Work out the finished part from the listing and answer in its coordinate system (mm). Face numbers are marked on the shaded views. A direction names the side the tool comes from. Coordinates: 2 decimals unless noted, no trailing zeros. Order: outer loops, then holes, each group sorted by start corner. A loop starts at its lowest first (then second) coordinate and runs counter-clockwise, first axis right, second up. Notation, with made-up numbers: M 65,3 L 107,3 A14 ccw 107,26 Z; hole C 16.25,-13 d10. An arc over 180 degrees is marked long. Use a Markdown table: item, result.
from build123d import *

# Parameters (mm, degrees)
BOSS_EXTRUDE1_DEPTH              = 25
SKETCH1_3_W                      = 34
SKETCH1_3_H                      = 9.5
SKETCH1_3_H_2                    = 24.5
BOSS_EXTRUDE2_DEPTH              = 30
F_6_6_6_6_DIAMETER_HOLE1_D       = 6.6
SKETCH4_R                        = 6
CUT_EXTRUDE1_DEPTH               = 30
F_10_8_10_8_DIAMETER_HOLE1_D     = 10.8
F_10_8_10_8_DIAMETER_HOLE1_DEPTH = 5
F_10_8_10_8_DIAMETER_HOLE1_TIP   = 3.244647343


with BuildPart() as part:
    # Sketch1 → Boss-Extrude1 (new body)
    with BuildSketch(Plane.XY):
        Polygon((-17, 16.25), (-30, 16.25), (-30, -16.25), (30, -16.25), (30, 16.25), (17, 16.25), (17, -8.25), (-17, -8.25), align=None)
    extrude(amount=BOSS_EXTRUDE1_DEPTH)

    # Sketch1_3 → Boss-Extrude2 (add)
    with BuildSketch(Plane.XY):
        with Locations((0, 21)):
            Rectangle(SKETCH1_3_W, SKETCH1_3_H)
        with Locations((0, 4)):
            Rectangle(SKETCH1_3_W, SKETCH1_3_H_2)
    extrude(amount=BOSS_EXTRUDE2_DEPTH)

    # 6.6 _6.6_ Diameter Hole1 (through all)
    with Locations(Plane(origin=(0, 16.25, 0), x_dir=(1, 0, 0), z_dir=(0, 1, 0))):
        with Locations((-23, -19), (-23, -6), (23, -6), (23, -19)):
            Hole(F_6_6_6_6_DIAMETER_HOLE1_D / 2)

    # Sketch4 → Cut-Extrude1 (cut)
    with BuildSketch(Plane.XY.offset(30)):
        with Locations((0, 8.75)):
            Circle(SKETCH4_R)
    extrude(amount=-CUT_EXTRUDE1_DEPTH, mode=Mode.SUBTRACT)

    # 10.8 _10.8_ Diameter Hole1
    with Locations(Plane(origin=(0, 16.25, 0), x_dir=(1, 0, 0), z_dir=(0, 1, 0))):
        with Locations((-23, -19), (-23, -6), (23, -6), (23, -19)):
            Hole(F_10_8_10_8_DIAMETER_HOLE1_D / 2, depth=F_10_8_10_8_DIAMETER_HOLE1_DEPTH)
            with Locations((0, 0, -(F_10_8_10_8_DIAMETER_HOLE1_DEPTH + F_10_8_10_8_DIAMETER_HOLE1_TIP / 2))):  # 118° drill point
                Cone(0, F_10_8_10_8_DIAMETER_HOLE1_D / 2, F_10_8_10_8_DIAMETER_HOLE1_TIP, mode=Mode.SUBTRACT)


solid = part.part
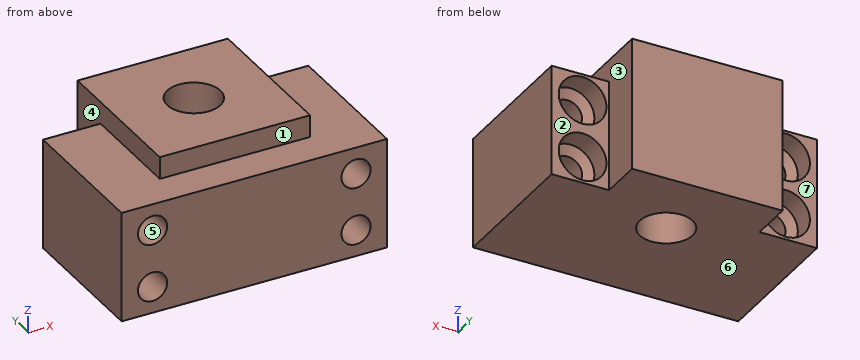
1. For a pull along Z with two mould halves and no side action, classify the marked faces 5, 6 and 7 as +Z half, -Z half, draft (parallel to the pull), parting line (faces both ways), or undercut.
Answers below:
| item | result |
|---|---|
| face 5 | undercut |
| face 6 | -Z half |
| face 7 | draft |
2. Section C-C on x = 0 is taken. Determine the outline of the cut face in (y, z), then the cut area to 3 significant figures.
Answers below:
| item | result |
|---|---|
| outline | M -16.25,0 L 2.75,0 L 2.75,30 L -8.25,30 L -8.25,25 L -16.25,25 Z; M 14.75,0 L 25.75,0 L 25.75,30 L 14.75,30 Z |
| area | 860 mm² |
3. For the marked faces 1, 2, 3 and 4, determine the directions among +Z, -Z, +X, -X, +Y, -Y from which every point of the face is accessible in a straight line to the end or side of a thin tool.
Answers below:
| item | result |
|---|---|
| face 1 | +Z, +X, -X, -Y |
| face 2 | +Z, -Z, +X, +Y |
| face 3 | +Z, +X, +Y |
| face 4 | +Z, -X, +Y |
4. Find the intervals of material crossed by probe 1 along Z at (x, y) = (-23, -9.75); probe 2 along Z at (x, y) = (-23, 14.7); probe 3 along X at (y, z) = (0, 19), in increasing order.
Answers below:
| item | result |
|---|---|
| probe 1 | 0 to 2.7, 9.3 to 15.7, 22.3 to 25 |
| probe 2 | 0 to 0.6, 11.4 to 13.6, 24.4 to 25 |
| probe 3 | -30 to -26.3, -19.7 to 19.7, 26.3 to 30 |
5. Flat-ended cylindrical pins translate along their axes: P1, Ø15, axis at y = 16.5, z = 15.5, coming from the -X side; P2, Ø6.5, axis at x = -21, z = 13.5, coming from the +Y side; P3, Ø8.5, axis at x = 23, z = 19, coming from the +Y side. Find the tip coordinate at first contact, or state that the pin passes through.
Answers below:
| item | result |
|---|---|
| P1 | x = -30 |
| P2 | y = 16.25 |
| P3 | y = 10.56 |
6. Section D-D on y = -10.5 is taken. Determine the outline of the cut face in (x, z).
Answers below:
| item | result |
|---|---|
| outline | M -30,0 L 30,0 L 30,25 L -30,25 Z; hole C -23,6 d6.6; hole C -23,19 d6.6; hole C 23,6 d6.6; hole C 23,19 d6.6 |
7. Section B-B on y = 7.5 is taken. Determine the outline of the cut face in (x, z).
Answers below:
| item | result |
|---|---|
| outline | M -30,0 L -5.87,0 L -5.87,30 L -17,30 L -17,25 L -30,25 Z; M 5.87,0 L 30,0 L 30,25 L 17,25 L 17,30 L 5.87,30 Z; hole C -23,6 d6.6; hole C -23,19 d6.6; hole C 23,6 d6.6; hole C 23,19 d6.6 |
8. Section A-A on z = 6 is taken. Determine the outline of the cut face in (x, y), then the cut area to 3 significant figures.
Answers below:
| item | result |
|---|---|
| outline | M -30,-16.25 L -26.3,-16.25 L -26.3,9.99 L -28.4,11.25 L -28.4,16.25 L -30,16.25 Z; M -19.7,-16.25 L 19.7,-16.25 L 19.7,9.99 L 17.6,11.25 L 17.6,16.25 L 17,16.25 L 17,25.75 L -17,25.75 L -17,16.25 L -17.6,16.25 L -17.6,11.25 L -19.7,9.99 Z; M 26.3,-16.25 L 30,-16.25 L 30,16.25 L 28.4,16.25 L 28.4,11.25 L 26.3,9.99 Z; hole C 0,8.75 d12 |
| area | 1,680 mm² |
